```python
from build123d import *

# Parameters (mm, degrees)
SKETCH_R         = 2.75
SKETCH_W         = 27.5
SKETCH_H         = 25
PAD_DEPTH        = 10
SKETCH001_W      = 30
SKETCH001_H      = 20
PAD001_DEPTH     = 30
PAD002_DEPTH     = 35
SKETCH003_W      = 20
SKETCH003_H      = 20
POCKET_DEPTH     = 15
SKETCH004_W      = 20
SKETCH004_H      = 15
POCKET001_DEPTH  = 64.000985
HOLE_D           = 5.5
HOLE_CBORE_D     = 9
HOLE_CBORE_DEPTH = 15
POCKET003_DEPTH  = 10.001
SKETCH011_W      = 30
SKETCH011_H      = 10
POCKET004_DEPTH  = 5
CHAMFER_SIZE     = 4.999
SKETCH012_R      = 2.25
HOLE001_DEPTH    = 10
SKETCH013_W      = 25
SKETCH013_H      = 21
POCKET005_DEPTH  = 10.001
SKETCH014_R      = 2.25
HOLE002_DEPTH    = 43.000985
SKETCH015_R      = 1.15
POCKET006_DEPTH  = 5
PAD003_DEPTH     = 10
CHAMFER001_SIZE  = 1
SKETCH017_R      = 1.25
HOLE003_DEPTH    = 10
HOLE003_TIPS_R   = 1.25
CHAMFER002_SIZE  = 1


with BuildPart() as part:
    # Sketch → Pad (new body)
    with BuildSketch(Plane.XY):
        with BuildLine():
            Line((100, 0), (100, 51.999985))
            ThreePointArc((100, 51.999985), (96.485281, 60.485267), (88, 63.999985))
            Line((12, 63.999985), (88, 63.999985))
            ThreePointArc((12, 63.999985), (3.514719, 60.485267), (0, 51.999985))
            Line((0, 51.999985), (0, 0))
            Line((0, 0), (100, 0))
        make_face()
        with Locations((12, 51.999985)):
            Circle(SKETCH_R, mode=Mode.SUBTRACT)
        with Locations((88, 51.999985)):
            Circle(SKETCH_R, mode=Mode.SUBTRACT)
        Polygon((32.5, 45), (32.5, 20), (5, 20), (5, 45), (18.75, 45), align=None, mode=Mode.SUBTRACT)
        with Locations((81.25, 32.5)):
            Rectangle(SKETCH_W, SKETCH_H, mode=Mode.SUBTRACT)
        with BuildLine():
            ThreePointArc((47.25, 9.499985), (50, 6.749985), (52.75, 9.499985))
            Line((52.75, 9.499985), (52.75, 14.499985))
            ThreePointArc((52.75, 14.499985), (50, 17.249985), (47.25, 14.499985))
            Line((47.25, 9.499985), (47.25, 14.499985))
        make_face(mode=Mode.SUBTRACT)
    extrude(amount=PAD_DEPTH)

    # Sketch001 (on Face23 of Pad) → Pad001 (join)
    with BuildSketch(Plane.XY.offset(10)):
        with Locations((23.5, 10)):
            Rectangle(SKETCH001_W, SKETCH001_H)
    extrude(amount=PAD001_DEPTH)

    # Sketch002 (on Face5 of Pad001) → Pad002 (join)
    with BuildSketch(Plane.XY.offset(10)):
        Polygon((63.5, 10), (57, 10), (57, 20), (100, 20), (100, 10), (93.5, 10), (93.5, 0), (63.5, 0), align=None)
    extrude(amount=PAD002_DEPTH)

    # Sketch003 (on Face9 of Pad002) → Pocket (cut)
    with BuildSketch(Plane.XZ):
        with Locations((23.5, 25)):
            Rectangle(SKETCH003_W, SKETCH003_H)
        with Locations((78.5, 25)):
            Rectangle(SKETCH003_W, SKETCH003_H)
    extrude(amount=-POCKET_DEPTH, mode=Mode.SUBTRACT)

    # Sketch004 (on Face9 of Pocket) → Pocket001 (cut, through all)
    with BuildSketch(Plane.XZ):
        with Locations((23.5, 25)):
            Rectangle(SKETCH004_W, SKETCH004_H)
        with Locations((78.5, 25)):
            Rectangle(SKETCH004_W, SKETCH004_H)
    extrude(amount=-POCKET001_DEPTH, mode=Mode.SUBTRACT)

    # Hole (through all)
    with Locations(Plane.XZ):
        with Locations((81.25, 5), (18.75, 5)):
            CounterBoreHole(HOLE_D / 2, HOLE_CBORE_D / 2, HOLE_CBORE_DEPTH)

    # Sketch010 → Pocket003 (cut, through all)
    with BuildSketch(Plane.XY.offset(10)):
        with BuildLine():
            ThreePointArc((47.748891, 59.001218), (44.998891, 61.751218), (42.248891, 59.001218))
            Line((42.248891, 59.001218), (42.248891, 54.001218))
            ThreePointArc((42.248891, 54.001218), (44.998891, 51.251218), (47.748891, 54.001218))
            Line((47.748891, 59.001218), (47.748891, 54.001218))
        make_face()
        with BuildLine():
            ThreePointArc((57.748891, 59.001218), (54.998891, 61.751218), (52.248891, 59.001218))
            Line((52.248891, 59.001218), (52.248891, 54.001218))
            ThreePointArc((52.248891, 54.001218), (54.998891, 51.251218), (57.748891, 54.001218))
            Line((57.748891, 59.001218), (57.748891, 54.001218))
        make_face()
    extrude(amount=-POCKET003_DEPTH, mode=Mode.SUBTRACT)

    # Sketch011 (on Face41 of Pocket003) → Pocket004 (cut)
    with BuildSketch(Plane.XY.offset(45)):
        with Locations((78.5, 5)):
            Rectangle(SKETCH011_W, SKETCH011_H)
    extrude(amount=-POCKET004_DEPTH, mode=Mode.SUBTRACT)

    # Chamfer
    chamfer_edges = [part.edges().sort_by_distance(p)[0] for p in [
        (60.25, 10, 45),
        (78.5, 10, 45),
        (96.75, 10, 45),
    ]]
    chamfer(chamfer_edges, length=CHAMFER_SIZE)

    # Sketch012 (on Face6 of Chamfer) → Hole001 (cut)
    with BuildSketch(Plane(origin=(0, 20, 0), x_dir=(-1, 0, 0), z_dir=(0, 1, 0))):
        with Locations((-94.25, 20)):
            Circle(SKETCH012_R)
        with Locations((-62.75, 20)):
            Circle(SKETCH012_R)
    extrude(amount=-HOLE001_DEPTH, mode=Mode.SUBTRACT)

    # Sketch013 (on Face15 of Hole001) → Pocket005 (cut, through all)
    with BuildSketch(Plane.XY.offset(10)):
        with Locations((50, 53.499985)):
            Rectangle(SKETCH013_W, SKETCH013_H)
    extrude(amount=-POCKET005_DEPTH, mode=Mode.SUBTRACT)

    # Sketch014 (on Face36 of Pocket005) → Hole002 (cut, through all)
    with BuildSketch(Plane(origin=(0, 42.999985, 0), x_dir=(-1, 0, 0), z_dir=(0, 1, 0))):
        with Locations((-56.25, 5)):
            Circle(SKETCH014_R)
        with Locations((-43.75, 5)):
            Circle(SKETCH014_R)
    extrude(amount=-HOLE002_DEPTH, mode=Mode.SUBTRACT)

    # Sketch015 (on Face55 of Hole002) → Pocket006 (cut)
    with BuildSketch(Plane(origin=(38.5, 0, 0), x_dir=(0, -1, 0), z_dir=(-1, 0, 0))):
        with Locations((-7.3, 34.85)):
            Circle(SKETCH015_R)
        with Locations((-7.3, 25.35)):
            Circle(SKETCH015_R)
    extrude(amount=POCKET006_DEPTH, mode=Mode.SUBTRACT)

    # Sketch016 (on Face15 of Pocket006) → Pad003 (join)
    with BuildSketch(Plane.XY.offset(10)):
        Polygon((100, 51.999985), (88, 63.999985), (100, 63.999985), align=None)
    extrude(amount=-PAD003_DEPTH)

    # Chamfer001
    chamfer001_edges = [part.edges().sort_by_distance(p)[0] for p in [
        (13.5, 0, 25),
        (13.5, 0, 33.75),
        (23.5, 0, 35),
        (13.5, 0, 16.25),
        (23.5, 0, 15),
        (33.5, 0, 25),
        (33.5, 0, 33.75),
        (33.5, 0, 16.25),
        (68.5, 0, 25),
        (68.5, 0, 16.25),
        (68.5, 0, 33.75),
        (78.5, 0, 35),
        (88.5, 0, 33.75),
        (88.5, 0, 25),
        (88.5, 0, 16.25),
        (78.5, 0, 15),
    ]]
    chamfer(chamfer001_edges, length=CHAMFER001_SIZE)

    # Sketch017 (on Face10 of Chamfer001) → Hole003 (cut)
    with BuildSketch(Plane.XZ):
        with Locations((50, 5)):
            Circle(SKETCH017_R)
    extrude(amount=-HOLE003_DEPTH, mode=Mode.SUBTRACT)

    # Hole003 tips → Hole003 tip 1 section 0
    with BuildSketch(Plane.XZ.offset(-10), mode=Mode.PRIVATE) as hole003_tip_1_s0:
        with Locations((50, 5)):
            Circle(HOLE003_TIPS_R)
    loft([hole003_tip_1_s0.sketch, Vertex(50, 10.751076, 5)], mode=Mode.SUBTRACT)

    # Chamfer002
    chamfer002_edges = [part.edges().sort_by_distance(p)[0] for p in [
        (51.25, 0, 5),
        (57, 17.4995, 45),
        (41.5, 42.999985, 5),
        (54, 42.999985, 5),
        (57, 12.4995, 42.5005),
    ]]
    chamfer(chamfer002_edges, length=CHAMFER002_SIZE)


solid = part.part
```
Could you check a few things on this model? Use its own coordinates, in mm. A direction names the side the tool comes from. Round coordinates to 2 decimals unless told otherwise and drop trailing zeros. Loops run counter-clockwise (first coordinate to the right, second up) from the corner with the lowest first, then second, coordinate; pieces in that order, holes last. Notation, with made-up numbers: (45.25, 6) -> (65.25, 6) arc R4 cw to (65.25, 11) -> close; hole circle Ø7 at (-0.75, -7). An arc over 180 degrees is marked (long way). One line per question, with ' | ' between items.
(1) For pin 1 Ø2 at (x, z) = (50, 5) entering from +Y; pin 2 Ø10 at (x, z) = (74, 37) entering from +Y; pin 3 Ø9 at (x, y) = (12, 52) entering from +Z, each with a flat end and sliding along its axis, tell me the tip position at first contact or that it passes through.
Model answer:
pin 1: stops at y = 43 | pin 2: stops at y = 20 | pin 3: stops at z = 10
(2) Thinking about a two-plate mould opening in Z: for faces 6 (the face through (23, 8, 15)), 7 (the face through (57.51, 12.45, 41.76)), 8 (the face through (50.06, 17.25, 4.93)), which applies, released by +Z, released by -Z, zero draft, split by the parting line, or undercut?
Model answer:
face 6: undercut | face 7: released by +Z | face 8: zero draft
(3) If we section it at A-A on x = 81.25: Count the separate pieces of the cut face and the enclosed holes in it, and give its area (3 significant figures).
Model answer:
separate pieces: 5 | enclosed holes: 0 | area: 385 mm^2
(4) For faces 1 (the face through (79, 15, 3)), 2 (the face through (57, 15, 27)), 3 (the face through (22, 20, 15)), 4 (the face through (23, 10, 40)), 5 (the face through (23, 17, 32.5)), which set-ups out of +Z, -Z, +X, -X, +Y, -Y let a thin tool reach every point of the face, with its end or its side?
Model answer:
face 1: -Y | face 2: +Z, +Y, -Y | face 3: +Z | face 4: +Z, -X, +Y, -Y | face 5: +Y, -Y
(5) If we section it at B-B on y = 28: List the corners of the cut face in (x, z) for me, and give its area (3 significant figures).
Model answer:
outline: (0, 0) -> (5, 0) -> (5, 10) -> (0, 10) -> close; (32.5, 0) -> (67.5, 0) -> (67.5, 10) -> (32.5, 10) -> close; (95, 0) -> (100, 0) -> (100, 10) -> (95, 10) -> close; hole circle Ø4.5 at (43.75, 5); hole circle Ø4.5 at (56.25, 5) | area: 418 mm^2
(6) If we section it at D-D on z = 12: List the corners of the cut face in (x, y) for me, and give its area (3 significant figures).
Model answer:
outline: (8.5, 0) -> (38.5, 0) -> (38.5, 20) -> (8.5, 20) -> close; (57, 10) -> (63.5, 10) -> (63.5, 0) -> (93.5, 0) -> (93.5, 10) -> (100, 10) -> (100, 20) -> (57, 20) -> close | area: 1,330 mm^2
(7) If we section it at C-C on x = 50: List the corners of the cut face in (y, z) for me, and give its area (3 significant figures).
Model answer:
outline: (0, 0) -> (6.75, 0) -> (6.75, 3.75) -> (1, 3.75) -> (0, 2.75) -> close; (0, 7.25) -> (1, 6.25) -> (6.75, 6.25) -> (6.75, 10) -> (0, 10) -> close; (17.25, 0) -> (43, 0) -> (43, 10) -> (17.25, 10) -> close | area: 307 mm^2
(8) If I drill on probe 1 along Z at (x, y) = (36.25, 7.3); probe 2 along Z at (x, y) = (18.75, 18.4); probe 3 along X at (y, z) = (8, 23), over which ranges is the centre line in solid material (lowest first)?
Model answer:
probe 1: z = 0 to 24.2, 26.5 to 33.7, 36 to 40 | probe 2: z = 0 to 2.25, 7.75 to 17.5, 32.5 to 40 | probe 3: x = 8.5 to 13.5, 33.5 to 38.5, 63.5 to 68.5, 88.5 to 93.5
